Input: part model. Units: mm. Frame: model coordinates. A direction names the side the tool comes from. Give positions to 0.01 mm unless a question says otherwise; leave off trailing zeros. Loops run counter-clockwise (first coordinate to the right, second up) from the corner with the lowest first, then second, coordinate; pieces in that order, holes last. Notation, with made-up numbers: M -19.5,-33.75 L 12.5,-33.75 A23 cw 12.5,-10.75 Z; hole C -28.5,-22.5 d5. An arc over 180 degrees is marked long. Use CSV: the item, a comma, the result in double quotes. Start each with the question number.
from build123d import *

# Parameters (mm, degrees)
SKETCH1_W           = 11.938
SKETCH1_H           = 11.938
BOSS_EXTRUDE1_DEPTH = 213.106
SKETCH2_R           = 3.68046
BOSS_EXTRUDE2_DEPTH = 22.225
SKETCH4_W           = 4.572
SKETCH4_H           = 4.572
BOSS_EXTRUDE4_DEPTH = 15.24
SKETCH5_R           = 13.051144527
CUT_EXTRUDE1_DEPTH  = 139.573
SKETCH6_W           = 7.62
SKETCH6_H           = 7.62
CUT_EXTRUDE2_DEPTH  = 12.7
SKETCH3_R           = 4.0005
CUT_EXTRUDE4_DEPTH  = 14.2875


with BuildPart() as part:
    # Sketch1 → Boss-Extrude1 (new body)
    with BuildSketch(Plane(origin=(0, 0, 0), x_dir=(1, 0, 0), z_dir=(0, 1, 0))):
        Rectangle(SKETCH1_W, SKETCH1_H)
    extrude(amount=BOSS_EXTRUDE1_DEPTH)

    # Sketch2 → Boss-Extrude2 (add)
    with BuildSketch(Plane(origin=(0, 213.106, 0), x_dir=(1, 0, 0), z_dir=(0, 1, 0))):
        Circle(SKETCH2_R)
    extrude(amount=BOSS_EXTRUDE2_DEPTH)

    # Sketch4 → Boss-Extrude4 (add)
    with BuildSketch(Plane(origin=(0, 235.331, 0), x_dir=(1, 0, 0), z_dir=(0, 1, 0))):
        Rectangle(SKETCH4_W, SKETCH4_H)
    extrude(amount=BOSS_EXTRUDE4_DEPTH)

    # Sketch5 → Cut-Extrude1 (cut)
    with BuildSketch(Plane(origin=(0, 250.571, 0), x_dir=(1, 0, 0), z_dir=(0, 1, 0))):
        Circle(SKETCH5_R)
    extrude(amount=-CUT_EXTRUDE1_DEPTH, mode=Mode.SUBTRACT)

    # Sketch6 → Cut-Extrude2 (cut)
    with BuildSketch(Plane(origin=(0, 110.998, 0), x_dir=(1, 0, 0), z_dir=(0, 1, 0))):
        Rectangle(SKETCH6_W, SKETCH6_H)
    extrude(amount=-CUT_EXTRUDE2_DEPTH, mode=Mode.SUBTRACT)

    # Sketch3 → Cut-Extrude4 (cut)
    with BuildSketch(Plane(origin=(0, 0, 0), x_dir=(-1, 0, 0), z_dir=(0, -1, 0))):
        Circle(SKETCH3_R)
    extrude(amount=-CUT_EXTRUDE4_DEPTH, mode=Mode.SUBTRACT)


solid = part.part
Item 1: Section A-A (x = 0). Output: boundary loops of the cut face in (y, z).
Item 2: Mould query, pull axis X, two halves, no side actions, for faces 1 (the flat face through (5.969, 55, 0)), 2 (the flat face through (0, 110.998, 4)), 3 (the flat face through (0, 14.288, 0)). Classes: +X half, -X half, draft (parallel to the pull), parting line (faces both ways), or undercut.
Item 3: Section B-B (z = 0). Output: boundary loops of the cut face in (x, y).
Item 4: Material intervals for line 1 (Z direction, x = 0, y = 10.5); line 2 (Z direction, x = 3, y = 106), sorted ascending.
Item 5: Set-up query: faces 4 (the cylindrical face through (0.9, 7, 3.9)), 5 (the flat face through (0, 55, -5.969)), 6 (the flat face through (-3.81, 105, 0)). Return all of +Z, -Z, +X, -X, +Y, -Y with unobstructed straight access to the full face (end or side cutting, diameter ignored); none if empty.
Item 6: First-contact query: pin 1 Ø7 at (x, z) = (0, 0) entering from +Y; pin 2 Ø4 at (x, z) = (-0.5, 1) entering from -Y. Flat tips, straight axial feed; report the tip coordinate or a pass-through.
Recorded:
1,outline,"M 0,-5.97 L 111,-5.97 L 111,-3.81 L 98.3,-3.81 L 98.3,3.81 L 111,3.81 L 111,5.97 L 0,5.97 L 0,4 L 14.29,4 L 14.29,-4 L 0,-4 Z"
2,face 1,"+X half"
2,face 2,"draft"
2,face 3,"undercut"
3,outline,"M -5.97,0 L -4,0 L -4,14.29 L 4,14.29 L 4,0 L 5.97,0 L 5.97,111 L 3.81,111 L 3.81,98.3 L -3.81,98.3 L -3.81,111 L -5.97,111 Z"
4,line 1,"-5.97 to -4, 4 to 5.97"
4,line 2,"-5.97 to -3.81, 3.81 to 5.97"
5,face 4,"-Y"
5,face 5,"-Z, +X, -X, +Y, -Y"
5,face 6,"+Y"
6,pin 1,"y = 98.3"
6,pin 2,"y = 14.29"
